The listing builds one solid part. Answer for the finished solid, in the listing's coordinates (mm). A direction names the side the tool comes from. Round coordinates to 2 decimals unless told otherwise and drop trailing zeros. Order: outer loops, then holes, each group sorted by start corner. A loop starts at its lowest first (then second) coordinate and runs counter-clockwise, first axis right, second up. Notation, with made-up numbers: (-32.5, 44.5) - (26.5, 44.5) arc R17 cw to (26.5, 56.5) - close; hole circle Ø11 at (81, -29). An arc over 180 degrees is marked (long way). Write item = value, one per line.
from build123d import *

# Parameters (mm, degrees)
SKETCH7_R            = 14.5
SKETCH7_R_2          = 12.5
BOSS_EXTRUDE2_DEPTH  = 4
BOSS_EXTRUDE6_START  = 3.5
SKETCH7_3_R          = 14.5
BOSS_EXTRUDE6_DEPTH  = 0.5
BOSS_EXTRUDE10_START = 4.3
BOSS_EXTRUDE10_DEPTH = 4.3
BOSS_EXTRUDE9_DEPTH  = 3
FILLET6_R            = 0.5
CUT_EXTRUDE1_DEPTH   = 58.25155
SKETCH16_R           = 1
BOSS_EXTRUDE11_DEPTH = 1
FILLET7_R            = 0.5
EXTRUDE_THIN2_START  = 3
SKETCH17_R           = 13.5
SKETCH17_R_2         = 12.5
EXTRUDE_THIN2_DEPTH  = 3


with BuildPart() as part:
    # Sketch7 → Boss-Extrude2 (new body)
    with BuildSketch(Plane(origin=(0, 0, 0), x_dir=(1, 0, 0), z_dir=(0, 1, 0))):
        with Locations(Location((40, 0, 0), (0, 0, 270))):
            Circle(SKETCH7_R)
        with Locations(Location((40, 0, 0), (0, 0, 270))):
            Circle(SKETCH7_R_2, mode=Mode.SUBTRACT)
    extrude(amount=BOSS_EXTRUDE2_DEPTH)

    # Sketch7_3 → Boss-Extrude6 (add)
    with BuildSketch(Plane(origin=(0, 0, 0), x_dir=(1, 0, 0), z_dir=(0, 1, 0)).offset(BOSS_EXTRUDE6_START)):
        with Locations(Location((40, 0, 0), (0, 0, 270))):
            Circle(SKETCH7_3_R)
    extrude(amount=BOSS_EXTRUDE6_DEPTH)

    # Sketch14 → Boss-Extrude10 (add)
    with BuildSketch(Plane.XZ.offset(-3.5).offset(BOSS_EXTRUDE10_START)):
        with BuildLine():
            Line((48.005623, -9.6), (31.994377, -9.6))
            ThreePointArc((31.994377, -9.6), (40, -12.5), (48.005623, -9.6))
        make_face()
        with BuildLine():
            Line((50.85, -6.207052), (50.85, 6.207052))
            ThreePointArc((50.85, 6.207052), (52.5, 0), (50.85, -6.207052))
        make_face()
        with BuildLine():
            Line((48.005623, 9.6), (31.994377, 9.6))
            ThreePointArc((31.994377, 9.6), (40, 12.5), (48.005623, 9.6))
        make_face()
        with BuildLine():
            Line((29.15, -6.207052), (29.15, 6.207052))
            ThreePointArc((29.15, 6.207052), (27.5, 0), (29.15, -6.207052))
        make_face()
    extrude(amount=-BOSS_EXTRUDE10_DEPTH)

    # Sketch11 → Boss-Extrude9 (add)
    with BuildSketch(Plane(origin=(0, 4, 0), x_dir=(1, 0, 0), z_dir=(0, 1, 0))):
        with BuildLine():
            Line((41.5, 17), (38.5, 17))
            Line((38.5, 17), (38.5, 13.919411))
            ThreePointArc((38.5, 13.919411), (40, 14), (41.5, 13.919411))
            Line((41.5, 13.919411), (41.5, 17))
        make_face()
        with BuildLine():
            ThreePointArc((41.5, -13.919411), (40, -14), (38.5, -13.919411))
            Line((38.5, -13.919411), (38.5, -17))
            Line((38.5, -17), (41.5, -17))
            Line((41.5, -17), (41.5, -13.919411))
        make_face()
    extrude(amount=-BOSS_EXTRUDE9_DEPTH)

    # Fillet6
    fillet6_edges = [part.edges().sort_by_distance(p)[0] for p in [
        (38.5, 1, -15.711103),
        (41.5, 1, -15.711103),
        (40, 1, -17),
        (40, 1, 17),
        (38.5, 1, 15.711103),
        (41.5, 1, 15.711103),
    ]]
    fillet(fillet6_edges, radius=FILLET6_R)

    # Sketch15 → Cut-Extrude1 (cut, through all)
    with BuildSketch(Plane(origin=(0, 3.5, 0), x_dir=(-1, 0, 0), z_dir=(0, -1, 0))):
        with BuildLine():
            ThreePointArc((-48.778949, 0.086066), (-48.086339, 0.115409), (-47.42595, -0.09544))
            Line((-47.42595, -0.09544), (-39.890389, 1.574116))
            Line((-39.890389, 1.574116), (-39.992029, 2.032869))
            Line((-39.992029, 2.032869), (-48.778949, 0.086066))
        make_face()
        with BuildLine():
            Line((-48.677309, -0.372687), (-47.42595, -0.09544))
            ThreePointArc((-47.42595, -0.09544), (-48.086339, 0.115409), (-48.778949, 0.086066))
            Line((-48.778949, 0.086066), (-48.677309, -0.372687))
        make_face()
        with BuildLine():
            ThreePointArc((-48.022691, -3.327313), (-49.827313, -2.177309), (-48.677309, -0.372687))
            Line((-48.677309, -0.372687), (-48.778949, 0.086066))
            ThreePointArc((-48.778949, 0.086066), (-50.286066, -2.278949), (-47.921051, -3.786066))
            Line((-47.921051, -3.786066), (-48.022691, -3.327313))
        make_face()
        with BuildLine():
            ThreePointArc((-47.921051, -3.786066), (-47.280863, -3.520118), (-46.771333, -3.050066))
            Line((-46.771333, -3.050066), (-48.022691, -3.327313))
            Line((-48.022691, -3.327313), (-47.921051, -3.786066))
        make_face()
        with BuildLine():
            Line((-39.235771, -1.380511), (-46.771333, -3.050066))
            ThreePointArc((-46.771333, -3.050066), (-47.280863, -3.520118), (-47.921051, -3.786066))
            Line((-47.921051, -3.786066), (-39.134131, -1.839264))
            Line((-39.134131, -1.839264), (-39.235771, -1.380511))
        make_face()
    extrude(amount=-CUT_EXTRUDE1_DEPTH, mode=Mode.SUBTRACT)

    # Sketch16 → Boss-Extrude11 (add)
    with BuildSketch(Plane(origin=(0, 3.5, 0), x_dir=(-1, 0, 0), z_dir=(0, -1, 0))):
        with Locations(Location((-48.35, -1.85, 0), (0, 0, 270))):
            Circle(SKETCH16_R)
    extrude(amount=BOSS_EXTRUDE11_DEPTH)

    # Fillet7
    fillet7_edges = [part.edges().sort_by_distance(p)[0] for p in [
        (48.35, 3.5, 0.85),
    ]]
    fillet(fillet7_edges, radius=FILLET7_R)

    # Sketch17 → Extrude-Thin2 (add)
    with BuildSketch(Plane(origin=(0, 0, 0), x_dir=(-1, 0, 0), z_dir=(0, -1, 0)).offset(EXTRUDE_THIN2_START)):
        with Locations((-40, 0)):
            Circle(SKETCH17_R)
        with Locations((-40, 0)):
            Circle(SKETCH17_R_2, mode=Mode.SUBTRACT)
    extrude(amount=-EXTRUDE_THIN2_DEPTH)


solid = part.part
Q1. Section B-B on x = 45 is taken. Determine the outline of the cut face in (y, z), then the cut area to 3 significant figures.
Model answer:
outline = (-3, -12.54) - (0, -12.54) - (0, -13.61) - (4, -13.61) - (4, -0.92) - (3.5, -0.92) - (3.5, -9.6) - (-0.8, -9.6) - (-0.8, -11.46) - (-3, -11.46) - close; (-3, 11.46) - (-0.8, 11.46) - (-0.8, 9.6) - (3.5, 9.6) - (3.5, 3.14) - (4, 3.14) - (4, 13.61) - (0, 13.61) - (0, 12.54) - (-3, 12.54) - close; (3.5, -0.44) - (4, -0.44) - (4, 2.66) - (3.5, 2.66) - close
area = 50.7 mm^2
Q2. Determine the mould class of faces 4 (the face through (40, 3, -17)), 5 (the face through (29.15, 1, 0)), 6 (the face through (40, 1, -9.6)), 7 (the face through (44.36, 1.97, 13.83)) for opening direction Z: released by +Z, released by -Z, zero draft, split by the parting line, or undercut.
Model answer:
face_4 = released by -Z
face_5 = undercut
face_6 = undercut
face_7 = split by the parting line
Q3. Flat-ended cylindrical pins translate along their axes: P1, Ø0.6, axis at x = 40, z = 15, coming from the -Y side; P2, Ø1.5, axis at y = -0.5, z = 3, coming from the -X side; P3, Ø3, axis at y = 2.5, z = -16, coming from the +X side. Find the tip coordinate at first contact, or state that the pin passes through.
Model answer:
P1 = 1
P2 = 25.71
P3 = 41.5
Q4. Section C-C on z = 7.5 is taken. Determine the outline of the cut face in (x, y).
Model answer:
outline = (27.59, 0) - (28.78, 0) - (28.78, -3) - (30, -3) - (30, 3.5) - (50, 3.5) - (50, -3) - (51.22, -3) - (51.22, 0) - (52.41, 0) - (52.41, 4) - (27.59, 4) - close
Q5. Section A-A on z = -0.5 is taken. Determine the outline of the cut face in (x, y), then the cut area to 3 significant figures.
Model answer:
outline = (25.51, 0) - (26.51, 0) - (26.51, -3) - (27.51, -3) - (27.51, -0.8) - (29.15, -0.8) - (29.15, 3.5) - (44.74, 3.5) - (44.74, 4) - (25.51, 4) - close; (46.91, 3.5) - (50.85, 3.5) - (50.85, -0.8) - (52.49, -0.8) - (52.49, -3) - (53.49, -3) - (53.49, 0) - (54.49, 0) - (54.49, 4) - (46.91, 4) - close
area = 47.5 mm^2
Q6. Find the intervals of material crossed by line 1 (X direction, y = -2.3, z = 0); line 2 (Z direction, x = 40, y = -1.7); line 3 (Z direction, x = 40, y = -0.6), in increasing order. Write a range as from..to.
Model answer:
line_1 = 26.5..27.5, 52.5..53.5
line_2 = -13.5..-12.5, 12.5..13.5
line_3 = -13.5..-9.6, 9.6..13.5
Q7. For faces 1 (the face through (41.5, 3, -16)), 2 (the face through (53.487, -1.521, -0.594)), 3 (the face through (38.5, 3, -16)), determine the directions among +Z, -Z, +X, -X, +Y, -Y from which every point of the face is accessible in a straight line to the end or side of a thin tool.
Model answer:
face_1 = -Z, +X, +Y, -Y
face_2 = -Y
face_3 = -Z, -X, +Y, -Y
Q8. Section D-D on x = 32.5 is taken. Determine the outline of the cut face in (y, z), then the cut area to 3 significant figures.
Model answer:
outline = (-3, -11.22) - (0, -11.22) - (0, -12.41) - (4, -12.41) - (4, 12.41) - (0, 12.41) - (0, 11.22) - (-3, 11.22) - (-3, 10) - (-0.8, 10) - (-0.8, 9.6) - (3.5, 9.6) - (3.5, -9.6) - (-0.8, -9.6) - (-0.8, -10) - (-3, -10) - close
area = 40.1 mm^2
